Design review of the part built by this model. Coordinates are the model's own, in mm. A direction names the side the tool comes from. Coordinates: 2 decimals unless noted, no trailing zeros. Write each loop counter-clockwise with the first axis right and the second up, starting at its lowest first coordinate (ties: lowest second). Pieces come first, ordered by that corner, then holes. Notation, with made-up numbers: M -17.75,-39.75 L 34.25,-39.75 A17 ccw 34.25,-22.75 Z; hole C -36.75,62 d7. An arc over 180 degrees is marked long. Write item = value, one per line.
```python
from build123d import *

# Parameters (mm, degrees)
F0_W     = 100
F0_H     = 40
F1_DEPTH = 10
F3_DEPTH = 10
F4_R     = 2
F5_DEPTH = 25
F6_R     = 4.5
F7_DEPTH = 5.7
F8_W     = 40
F8_H     = 3
F9_DEPTH = 40.001
F10_R    = 5


with BuildPart() as f1:
    # F0 (on Top) → F1 (new body)
    with BuildSketch(Plane.XY):
        with Locations((-50, 20)):
            Rectangle(F0_W, F0_H)
    extrude(amount=F1_DEPTH)

    # F2 (on face) → F3 (join)
    with BuildSketch(Plane(origin=(0, 40, 0), x_dir=(-1, 0, 0), z_dir=(0, 1, 0))):
        with BuildLine():
            Line((30, 35), (30, 0))
            Line((30, 0), (70, 0))
            Line((70, 0), (70, 35))
            ThreePointArc((70, 35), (50, 55), (30, 35))
        make_face()
    extrude(amount=-F3_DEPTH)

    # F4 (on face) → F5 (cut)
    with BuildSketch(Plane(origin=(0, 40, 0), x_dir=(-1, 0, 0), z_dir=(0, 1, 0))):
        with Locations((50, 35)):
            Circle(F4_R)
    extrude(amount=-F5_DEPTH, mode=Mode.SUBTRACT)

    # F6 (on face) → F7 (cut)
    with BuildSketch(Plane(origin=(0, 40, 0), x_dir=(-1, 0, 0), z_dir=(0, 1, 0))):
        with Locations((50, 35)):
            Circle(F6_R)
    extrude(amount=-F7_DEPTH, mode=Mode.SUBTRACT)

    # F8 (on face) → F9 (cut, through all)
    with BuildSketch(Plane(origin=(0, 40, 0), x_dir=(-1, 0, 0), z_dir=(0, 1, 0))):
        with Locations((50, 1.5)):
            Rectangle(F8_W, F8_H)
    extrude(amount=-F9_DEPTH, mode=Mode.SUBTRACT)

    # F10
    f10_edges = [f1.edges().sort_by_distance(p)[0] for p in [
        (-70, 30, 22.5),
        (-30, 30, 22.5),
    ]]
    fillet(f10_edges, radius=F10_R)


solid = f1.part
```
Q1. Wall thickness on line 1 (Z direction, x = -50, y = 38.8); line 2 (Y direction, x = -59.5, z = 38); line 3 (Z direction, x = -54, y = 17): over which ranges is each line inside the solid? List them lowest first.
Check result:
line_1 = 3 to 30.5, 39.5 to 55
line_2 = 30 to 40
line_3 = 3 to 10
Q2. Consider section D-D, the plane z = 25. State the section outline as (x, y) points.
Check result:
outline = M -70,35 A5 ccw -65,30 L -35,30 A5 ccw -30,35 L -30,40 L -70,40 Z
Q3. For P1, Ø1.5, axis at x = -61, z = 21, coming from the -Y side; P2, Ø3.5, axis at x = -50, z = 35, coming from the -Y side; P3, Ø8, axis at x = -47, y = 6, coming from the -Z side; P4, Ø5.5, axis at y = 37, z = 27, coming from the -X side, all flat-tipped, find the tip position at first contact; note any pin that passes through.
Check result:
P1 = 30
P2 = through
P3 = 3
P4 = -70
Q4. Consider section A-A, the plane x = -50. State the section outline as (y, z) points, and give its area (3 significant figures).
Check result:
outline = M 0,3 L 40,3 L 40,30.5 L 34.3,30.5 L 34.3,33 L 30,33 L 30,10 L 0,10 Z; M 30,37 L 34.3,37 L 34.3,39.5 L 40,39.5 L 40,55 L 35,55 A5 ccw 30,50 Z
area = 656 mm²
Q5. Machinability: for faces 4 (the cylindrical face through (-32, 31, 22)), 5 (the cylindrical face through (-52.08, 37.19, 31.01)), 6 (the cylindrical face through (-68, 31, 23)), 7 (the flat face through (-30, 20, 1)), which of the approach directions +Z, -Z, +X, -X, +Y, -Y give a long, thin tool a straight path to every point of the face, cutting with its end or side? Answer none if there is none.
Check result:
face_4 = +Z, +X, -Y
face_5 = +Y
face_6 = +Z, -X, -Y
face_7 = -Z, +Y, -Y
Q6. Consider section B-B, the plane y = 37.5. State the section outline as (x, z) points.
Check result:
outline = M -100,0 L -70,0 L -70,3 L -30,3 L -30,0 L 0,0 L 0,10 L -30,10 L -30,35 A20 ccw -70,35 L -70,10 L -100,10 Z; hole C -50,35 d9
Q7. Consider section C-C, the plane y = 6. State the section outline as (x, z) points.
Check result:
outline = M -100,0 L -70,0 L -70,3 L -30,3 L -30,0 L 0,0 L 0,10 L -100,10 Z
Q8. The part is to be moulded in two halves that separate along Z. For faces 1 (the flat face through (0, 20, 5)), 2 (the flat face through (-51, 20, 10)), 3 (the cylindrical face through (-50.923, 32.18, 33.226)), say which applies: +Z half, -Z half, draft (parallel to the pull), parting line (faces both ways), or undercut.
Check result:
face_1 = draft
face_2 = +Z half
face_3 = undercut
